Could you check a few things on this model? Use its own coordinates, in mm. A direction names the side the tool comes from. Coordinates: 2 decimals unless noted, no trailing zeros. Loops run counter-clockwise (first coordinate to the right, second up) from the corner with the lowest first, then second, coordinate; pieces in that order, holes last.
from build123d import *

# Parameters (mm, degrees)
BOSS_EXTRUDE1_DEPTH  = 4.7625
M4_CLEARANCE_HOLE1_D = 4.5
SKETCH4_R            = 3.3
SKETCH4_R_2          = 2.9765625
SKETCH4_R_3          = 6.125
SKETCH4_R_4          = 11.9
CUT_EXTRUDE1_DEPTH   = 4.7625
BOSS_EXTRUDE3_DEPTH  = 4.7625
M4_CLEARANCE_HOLE2_D = 4.5


with BuildPart() as part:
    # Sketch1 → Boss-Extrude1 (new body)
    with BuildSketch(Plane.XY):
        with BuildLine():
            Line((50.349976536, 7.779015878), (19.528151129, 7.779015878))
            Line((19.528151129, 7.779015878), (16.547693582, 10.759473425))
            ThreePointArc((16.547693582, 10.759473425), (8.769518989, 10.759473425), (8.769518989, 2.981298831))
            Line((8.769518989, 2.981298831), (11.749976536, 0.000841285))
            Line((11.749976536, 0.000841285), (11.749976536, -43.901984122))
            Line((11.749976536, -43.901984122), (8.340276536, -43.901984122))
            ThreePointArc((8.340276536, -43.901984122), (2.840276536, -49.401984122), (8.340276536, -54.901984122))
            Line((8.340276536, -54.901984122), (11.749976536, -54.901984122))
            Line((11.749976536, -54.901984122), (11.749976536, -100.289984122))
            Line((11.749976536, -100.289984122), (8.340276536, -100.289984122))
            ThreePointArc((8.340276536, -100.289984122), (2.840276536, -105.789984122), (8.340276536, -111.289984122))
            Line((8.340276536, -111.289984122), (11.749976536, -111.289984122))
            Line((11.749976536, -111.289984122), (11.749976536, -155.192809529))
            Line((11.749976536, -155.192809529), (8.769518989, -158.173267075))
            ThreePointArc((8.769518989, -158.173267075), (8.769518989, -165.951441668), (16.547693582, -165.951441668))
            Line((16.547693582, -165.951441668), (19.528151129, -162.970984122))
            Line((19.528151129, -162.970984122), (50.349976536, -162.970984122))
            Line((50.349976536, -162.970984122), (50.349976536, -166.380684122))
            ThreePointArc((50.349976536, -166.380684122), (55.849976536, -171.880684122), (61.349976536, -166.380684122))
            Line((61.349976536, -166.380684122), (61.349976536, -162.970984122))
            Line((61.349976536, -162.970984122), (92.171801943, -162.970984122))
            Line((92.171801943, -162.970984122), (95.152259489, -165.951441668))
            ThreePointArc((95.152259489, -165.951441668), (102.930434082, -165.951441668), (102.930434082, -158.173267075))
            Line((102.930434082, -158.173267075), (99.949976536, -155.192809529))
            Line((99.949976536, -155.192809529), (99.949976536, -111.289984122))
            Line((99.949976536, -111.289984122), (103.359676536, -111.289984122))
            ThreePointArc((103.359676536, -111.289984122), (108.859676536, -105.789984122), (103.359676536, -100.289984122))
            Line((103.359676536, -100.289984122), (99.949976536, -100.289984122))
            Line((99.949976536, -100.289984122), (99.949976536, -54.901984122))
            Line((99.949976536, -54.901984122), (103.359676536, -54.901984122))
            ThreePointArc((103.359676536, -54.901984122), (108.859676536, -49.401984122), (103.359676536, -43.901984122))
            Line((103.359676536, -43.901984122), (99.949976536, -43.901984122))
            Line((99.949976536, -43.901984122), (99.949976536, 0.000841285))
            Line((99.949976536, 0.000841285), (102.930434082, 2.981298831))
            ThreePointArc((102.930434082, 2.981298831), (102.930434082, 10.759473425), (95.152259489, 10.759473425))
            Line((95.152259489, 10.759473425), (92.171801943, 7.779015878))
            Line((92.171801943, 7.779015878), (61.349976536, 7.779015878))
            Line((61.349976536, 7.779015878), (61.349976536, 11.188715878))
            ThreePointArc((61.349976536, 11.188715878), (55.849976536, 16.688715878), (50.349976536, 11.188715878))
            Line((50.349976536, 11.188715878), (50.349976536, 7.779015878))
        make_face()
    extrude(amount=-BOSS_EXTRUDE1_DEPTH)

    # M4 Clearance Hole1 (through all)
    with Locations(Plane(origin=(0, 0, -4.7625), x_dir=(-1, 0, 0), z_dir=(0, 0, -1))):
        with Locations((-12.658606286, -162.062354372), (-55.849976536, -166.380684122), (-99.041346785, -162.062354372), (-103.359676536, -105.789984122), (-103.359676536, -49.401984122), (-99.041346785, 6.870386128), (-12.658606286, 6.870386128), (-8.340276536, -49.401984122), (-8.340276536, -105.789984122), (-55.849976536, 11.188715878)):
            Hole(M4_CLEARANCE_HOLE1_D / 2)

    # Sketch4 → Cut-Extrude1 (cut)
    with BuildSketch(Plane(origin=(0, 0, -4.7625), x_dir=(-1, 0, 0), z_dir=(0, 0, -1))):
        with Locations((-41.616084767, -16.665859852)):
            Circle(SKETCH4_R)
        with Locations((-70.083868304, -40.3002691)):
            Circle(SKETCH4_R)
        with Locations((-27.909976536, -139.508484122)):
            Circle(SKETCH4_R_2)
        with Locations((-41.616084767, -76.466699143)):
            Circle(SKETCH4_R)
        with Locations((-83.789976536, -139.508484122)):
            Circle(SKETCH4_R_2)
        with Locations((-70.083868304, -100.101108391)):
            Circle(SKETCH4_R)
        with Locations((-66.009976536, -139.508484122)):
            Circle(SKETCH4_R_3)
        with Locations((-82.519976536, -59.220984122)):
            Circle(SKETCH4_R_3)
        with Locations((-45.689976536, -139.508484122)):
            Circle(SKETCH4_R_3)
        with Locations((-55.849976536, -88.283903767)):
            Circle(SKETCH4_R_4)
        with Locations((-55.849976536, -28.483064476)):
            Circle(SKETCH4_R_4)
    extrude(amount=-CUT_EXTRUDE1_DEPTH, mode=Mode.SUBTRACT)

    # Sketch6 → Boss-Extrude3 (add)
    with BuildSketch(Plane.XY):
        with BuildLine():
            Line((39.939063832, 7.779015878), (39.939063832, 12.779015878))
            ThreePointArc((39.939063832, 12.779015878), (34.939063832, 17.779015878), (29.939063832, 12.779015878))
            Line((29.939063832, 12.779015878), (29.939063832, 7.779015878))
            Line((29.939063832, 7.779015878), (39.939063832, 7.779015878))
        make_face()
        with BuildLine():
            Line((81.760889239, -162.970984122), (71.760889239, -162.970984122))
            Line((71.760889239, -162.970984122), (71.760889239, -167.970984122))
            ThreePointArc((71.760889239, -167.970984122), (76.760889239, -172.970984122), (81.760889239, -167.970984122))
            Line((81.760889239, -167.970984122), (81.760889239, -162.970984122))
        make_face()
    boss_extrude3 = extrude(amount=-BOSS_EXTRUDE3_DEPTH)

    # M4 Clearance Hole2 (through all)
    with Locations(Plane.XY):
        with Locations((34.939063832, 12.779015878), (76.760889239, -167.970984122)):
            m4_clearance_hole2 = Hole(M4_CLEARANCE_HOLE2_D / 2)

    # Mirror1: Boss-Extrude3, M4 Clearance Hole2 across plane
    add(boss_extrude3.mirror(Plane.ZY.offset(-55.849976536)))
    add(m4_clearance_hole2.mirror(Plane.ZY.offset(-55.849976536)), mode=Mode.SUBTRACT)


solid = part.part
(1) I need wall thicknesses on probe 1 along Y at (x, z) = (12.5, -2.9); probe 2 along Y at (x, z) = (48, -1.5); probe 3 along Y at (x, z) = (101.5, -0.45). Which ranges of each line are inside material? Lowest first, please.
Answers:
probe 1: y = -167.56 to -164.31, -159.82 to 4.63, 9.11 to 12.37
probe 2: y = -162.97 to -145.18, -133.84 to -97.23, -79.34 to -37.43, -19.54 to 7.78
probe 3: y = -166.98 to -156.74, -111.29 to -107.06, -104.52 to -100.29, -54.9 to -50.67, -48.14 to -43.9, 1.55 to 11.79
(2) We'd pull the mould along Y, two halves only. Please class faces 5 (the face through (76.65, -172.97, -2.35)), 6 (the face through (71.761, -165, -2)), 7 (the face through (10, -54.902, -2)): +Y half, -Y half, draft (parallel to the pull), parting line (faces both ways), or undercut.
Answers:
face 5: -Y half
face 6: draft
face 7: undercut
(3) Imagine slicing it at D-D, the plane z = -3.4. State how many separate pieces and enclosed holes the cut face has, and give its area (3 significant figures).
Answers:
separate pieces: 1
enclosed holes: 25
area: 14,500 mm2
(4) Imagine slicing it at C-C, the plane x = 21.5. Write out the boundary of the cut face in (y, z).
Answers:
outline: (-162.97, -4.76) - (7.78, -4.76) - (7.78, 0) - (-162.97, 0) - close
(5) Imagine slicing it at B-B, the plane y = -149.5. Write out the boundary of the cut face in (x, z).
Answers:
outline: (11.75, -4.76) - (99.95, -4.76) - (99.95, 0) - (11.75, 0) - close
(6) Imagine slicing it at A-A, the plane x = 56. Write out the boundary of the cut face in (y, z), and give its area (3 significant figures).
Answers:
outline: (-171.88, -4.76) - (-168.63, -4.76) - (-168.63, 0) - (-171.88, 0) - close; (-164.14, -4.76) - (-100.18, -4.76) - (-100.18, 0) - (-164.14, 0) - close; (-76.38, -4.76) - (-40.38, -4.76) - (-40.38, 0) - (-76.38, 0) - close; (-16.58, -4.76) - (8.94, -4.76) - (8.94, 0) - (-16.58, 0) - close; (13.43, -4.76) - (16.69, -4.76) - (16.69, 0) - (13.43, 0) - close
area: 629 mm2
(7) For pin 1 (11 mm diameter, centred on x = 66.01, y = -139.51, fed in from +Z); pin 2 (7 mm diameter, centred on x = 76.76, y = 12.78, fed in from -Z); pin 3 (1.4 mm diameter, centred on x = 45.5, z = -2.5, fed in from -Y); pin 4 (1.4 mm diameter, centred on y = 11, z = -2.5, fed in from -X), each with a flat end and sliding along its axis, tell me the tip position at first contact or that it passes through.
Answers:
pin 1: passes through
pin 2: stops at z = -4.76
pin 3: stops at y = -162.97
pin 4: stops at x = 8.36
(8) Which directions (+Z, -Z, +X, -X, +Y, -Y) give clear straight access to the entire face, cutting with the end or side of a thin tool? Please do faces 1 (the face through (11.75, -22, -2)), 2 (the face through (61.35, -165, -2)), 3 (the face through (28.297, -136.557, -2.415)), 4 (the face through (29.939, 10, -2)).
Answers:
face 1: +Z, -Z, -X
face 2: +Z, -Z, -Y
face 3: +Z, -Z
face 4: +Z, -Z, +Y
